Input: part model. Units: mm. Frame: model coordinates. Face numbers are marked on the shaded views. A direction names the side the tool comes from. Coordinates: 2 decimals unless noted, no trailing zeros. Order: outer loops, then holes, each group sorted by start corner. A loop starts at its lowest first (then second) coordinate and runs counter-clockwise, first axis right, second up. Notation, with made-up numbers: (68, 19.25) -> (111, 19.25) arc R36 ccw to (111, 58.25) -> close; hole circle Ø5 at (59.25, 41). An arc over 180 degrees is marked (long way). Write each question's results on one line, items separated by ' | '.
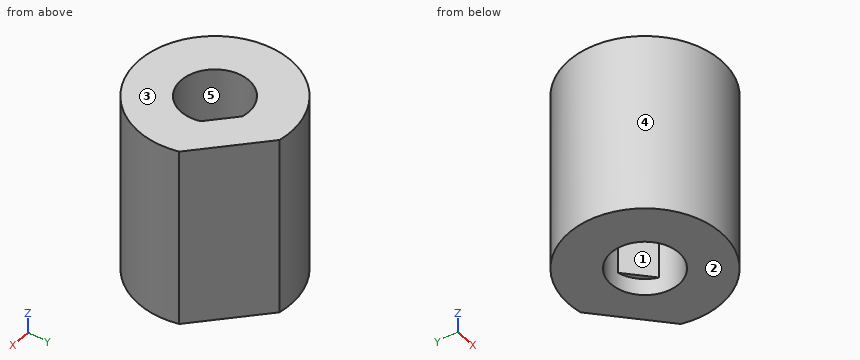
```python
from build123d import *

# Parameters (mm, degrees)
F1_DEPTH = 35
F2_R     = 6.604
F3_DEPTH = 38.1
F5_DEPTH = 31.75


# Not quite as in the source:
# - a feature names something its author has since deleted; it is built from what else it names


with BuildPart() as f1:
    # F0 (on Top) → F1 (new body)
    with BuildSketch(Plane.XY):
        with BuildLine():
            Line((14.3630077291, 3.7718044718), (2.6000410284, 14.6206117058))
            ThreePointArc((2.6000410284, 14.6206117058), (-10.0677907401, -10.9161389517), (14.3630077291, 3.7718044718))
        make_face()
    extrude(amount=F1_DEPTH)

    # F2 (on face) → F3 (cut)
    with BuildSketch(Plane.XY.offset(35)):
        Circle(F2_R)
    extrude(amount=-F3_DEPTH, mode=Mode.SUBTRACT)

    # F4 (on face) → F5 (join)
    with BuildSketch(Plane.XY.offset(35)):
        with BuildLine():
            ThreePointArc((6.3047218477, 1.9655275177), (4.4772855251, 4.854557686), (1.4501641617, 6.4428130428))
            Line((1.4501641617, 6.4428130428), (6.3047218477, 1.9655275177))
        make_face()
    extrude(amount=-F5_DEPTH)


solid = f1.part
```
(1) Mould query, pull axis X, two halves, no side actions, for the marked faces 3, 4 and 5. Classes: +X half, -X half, draft (parallel to the pull), parting line (faces both ways), or undercut.
Return value:
face 3: draft | face 4: parting line | face 5: undercut
(2) Pin query (flat end, axial travel): P1, Ø8, axis at x = -9.5, z = 12, coming from the -Y side; P2, Ø2, axis at x = 5.5, z = 9.5, coming from the -Y side; P3, Ø3, axis at y = -2.5, z = 24.5, coming from the +X side. Return the tip coordinate at first contact, or that it passes through.
Return value:
P1: y = -13.79 | P2: y = -14.15 | P3: x = 14.82
(3) Cut plane D-D, the plane y = 5.25. Return loops of the section in (x, z), plus the area to 3 significant figures.
Return value:
outline: (-13.89, 0) -> (-4.01, 0) -> (-4.01, 35) -> (-13.89, 35) -> close; (2.74, 3.25) -> (4.01, 3.25) -> (4.01, 0) -> (12.76, 0) -> (12.76, 35) -> (2.74, 35) -> close | area: 692 mm2
(4) Reachability of the marked faces 1 and 2 from +Z, -Z, +X, -X, +Y, -Y: full face, straight path, thin tool, end or side. Return the list, or none.
Return value:
face 1: +Z, -Z | face 2: -Z, +X, -X, +Y, -Y
(5) Line query: line 1 along X through (y, z) = (0, 13); line 2 along X through (y, z) = (6, 20). Output: solid intervals per line, ascending. Write a range as from..to.
Return value:
line 1: -14.85..-6.6, 6.6..14.85 | line 2: -13.58..-2.76, 1.93..11.95
(6) Cut plane C-C, the plane z = 25.5. Return loops of the section in (x, y).
Return value:
outline: (2.6, 14.62) arc R14.85 ccw (long way) to (14.36, 3.77) -> close; hole (1.45, 6.44) arc R6.6 ccw (long way) to (6.3, 1.97) -> close
(7) Cut plane A-A, the plane y = 0. Return loops of the section in (x, z).
Return value:
outline: (-14.85, 0) -> (-6.6, 0) -> (-6.6, 35) -> (-14.85, 35) -> close; (6.6, 0) -> (14.85, 0) -> (14.85, 35) -> (6.6, 35) -> close
